Design review of the part built by this model. Coordinates are the model's own, in mm. A direction names the side the tool comes from. Coordinates: 2 decimals unless noted, no trailing zeros. Loops run counter-clockwise (first coordinate to the right, second up) from the corner with the lowest first, then second, coordinate; pieces in that order, holes last. Notation, with made-up numbers: M 84,75 L 107,75 A17 cw 107,82 Z; hole C 8,-19 d1. An arc over 180 degrees is marked long. Answer as CSV lines item,"result". Start each with the question number.
from build123d import *

# Parameters (mm, degrees)
SKETCH009_W             = 84
SKETCH009_H             = 70
PAD002_DEPTH            = 2
SKETCH010_W             = 2
SKETCH010_H             = 7
PAD003_DEPTH            = 2
SKETCH012_W             = 8
SKETCH012_H             = 6.8
PAD004_DEPTH            = 4
SKETCH013_W             = 7
SKETCH013_H             = 6
PAD005_DEPTH            = 4
SKETCH011_W             = 8
SKETCH011_H             = 6.8
PAD006_DEPTH            = 4
SKETCH014_R             = 1.15
POCKET002_DEPTH         = 81.001
SKETCH016_R             = 1.15
POCKET003_DEPTH         = 8.501
SKETCH018_W             = 11.5
SKETCH018_H             = 11.5
POCKET004_DEPTH         = 5
POCKET005_DEPTH         = 5
POCKET006_DEPTH         = 5
SKETCH021_W             = 1
SKETCH021_H             = 7
PAD007_DEPTH            = 1
SKETCH022_W             = 9
SKETCH022_H             = 10
POCKET007_DEPTH         = 0.4
FILLET_R                = 3
BODY002_PITCH_ANGLE     = -90
BODY002_PLACEMENT_ANGLE = 90
PAD001_DEPTH            = 35
SKETCH007_W             = 11.5
SKETCH007_H             = 11.5
POCKET001_DEPTH         = 13
FILLET001_R             = 3
SKETCH025_W             = 6.5
SKETCH025_H             = 9
SKETCH025_W_2           = 9
SKETCH025_H_2           = 6.5
POCKET008_DEPTH         = 8


with BuildPart() as back:
    # Sketch009 → Pad002 (new body)
    with BuildSketch(Plane.XY):
        Rectangle(SKETCH009_W, SKETCH009_H)
    extrude(amount=PAD002_DEPTH)

    # Sketch010 (on Face6 of Pad002) → Pad003 (join)
    with BuildSketch(Plane.XY.offset(2)):
        with Locations((-38, -1)):
            Rectangle(SKETCH010_W, SKETCH010_H)
        Polygon((-21, 32), (39, 32), (39, -4), (37, -4), (37, 30), (-21, 30), align=None)
    extrude(amount=PAD003_DEPTH)

    # Sketch012 (on Face15 of Pad003) → Pad004 (join)
    with BuildSketch(Plane.YZ.offset(39)):
        with Locations((0, 5.4)):
            Rectangle(SKETCH012_W, SKETCH012_H)
    extrude(amount=-PAD004_DEPTH)

    # Sketch013 (on Face9 of Pad004) → Pad005 (join)
    with BuildSketch(Plane(origin=(-39, 0, 0), x_dir=(0, -1, 0), z_dir=(-1, 0, 0))):
        with Locations((1, 5)):
            Rectangle(SKETCH013_W, SKETCH013_H)
    extrude(amount=-PAD005_DEPTH)

    # Sketch011 (on Face16 of Pad003) → Pad006 (join)
    with BuildSketch(Plane(origin=(0, 32, 0), x_dir=(-1, 0, 0), z_dir=(0, 1, 0))):
        with Locations((-29, 5.4)):
            Rectangle(SKETCH011_W, SKETCH011_H)
        with Locations((14, 5.4)):
            Rectangle(SKETCH011_W, SKETCH011_H)
    extrude(amount=-PAD006_DEPTH)

    # Sketch014 (on Face44 of Pad006) → Pocket002 (cut, through all)
    with BuildSketch(Plane.YZ.offset(39)):
        with Locations((0, 5)):
            Circle(SKETCH014_R)
    extrude(amount=-POCKET002_DEPTH, mode=Mode.SUBTRACT)

    # Sketch016 → Pocket003 (cut, through all)
    with BuildSketch(Plane.XZ.offset(-26.5)):
        with Locations((-13, 5)):
            Circle(SKETCH016_R)
        with Locations((30, 5)):
            Circle(SKETCH016_R)
    extrude(amount=-POCKET003_DEPTH, mode=Mode.SUBTRACT)

    # Sketch018 (on Face5 of Pocket003) → Pocket004 (cut)
    with BuildSketch(Plane.XY.offset(2)):
        with Locations((0, 17.75)):
            Rectangle(SKETCH018_W, SKETCH018_H)
    extrude(amount=-POCKET004_DEPTH, mode=Mode.SUBTRACT)

    # Sketch019 (on Face31 of Pocket004) → Pocket005 (cut)
    with BuildSketch(Plane.XZ.offset(-28)):
        Polygon((29.125944, 9.042901), (33.258869, 4.499726), (33.258869, 9.042901), align=None)
    extrude(amount=-POCKET005_DEPTH, mode=Mode.SUBTRACT)

    # Sketch020 (on Face36 of Pocket005) → Pocket006 (cut)
    with BuildSketch(Plane(origin=(35, 0, 0), x_dir=(0, -1, 0), z_dir=(-1, 0, 0))):
        Polygon((2.77547, 8.938441), (6.386171, 3.079567), (6.386171, 8.938441), align=None)
    extrude(amount=-POCKET006_DEPTH, mode=Mode.SUBTRACT)

    # Sketch021 (on Face40 of Pocket006) → Pad007 (join)
    with BuildSketch(Plane.XY.offset(8)):
        with Locations((-38.5, -1)):
            Rectangle(SKETCH021_W, SKETCH021_H)
    extrude(amount=PAD007_DEPTH)

    # Sketch022 (on Face5 of Pocket005) → Pocket007 (cut)
    with BuildSketch(Plane.XY.offset(2)):
        with Locations((-30.3, 30)):
            Rectangle(SKETCH022_W, SKETCH022_H)
    extrude(amount=-POCKET007_DEPTH, mode=Mode.SUBTRACT)

    # Fillet
    fillet_edges = [back.edges().sort_by_distance(p)[0] for p in [
        (42, 35, 1),
        (-42, 35, 1),
    ]]
    fillet(fillet_edges, radius=FILLET_R)


with BuildPart() as back_1:
    # Body002 pitch: moved
    add(back.part.rotate(Axis((0, 0, 0), (0, 1, 0)), BODY002_PITCH_ANGLE))


with BuildPart() as back_2:
    # Body002 placement: moved
    add(back_1.part.rotate(Axis((0, 0, 0), (0, 0, 1)), BODY002_PLACEMENT_ANGLE))


with BuildPart() as curve:
    # Sketch006 → Pad001 (new body, symmetric)
    with BuildSketch(Plane(origin=(0, 0, 0), x_dir=(0, 0, -1), z_dir=(1, 0, 0))):
        with BuildLine():
            ThreePointArc((-42, 3.4), (0, 0.674728), (42, 3.4))
            Line((42, -0.1), (42, 3.4))
            Line((-42, -0.1), (42, -0.1))
            Line((-42, 3.4), (-42, -0.1))
        make_face()
    extrude(amount=PAD001_DEPTH, both=True)

    # Sketch007 (on Face3 of Pad001) → Pocket001 (cut)
    with BuildSketch(Plane.XZ.offset(0.1)):
        with Locations((-17.75, 0)):
            Rectangle(SKETCH007_W, SKETCH007_H)
    extrude(amount=-POCKET001_DEPTH, mode=Mode.SUBTRACT)

    # Fillet001
    fillet001_edges = [curve.edges().sort_by_distance(p)[0] for p in [
        (-35, 1.65, -42),
        (-35, 1.65, 42),
    ]]
    fillet(fillet001_edges, radius=FILLET001_R)

    # Boolean: union Back
    add(back_2.part)

    # Sketch025 (on Face32 of Boolean) → Pocket008 (cut, symmetric)
    with BuildSketch(Plane.XZ.offset(2)):
        with Locations((-28.75, 0)):
            Rectangle(SKETCH025_W, SKETCH025_H)
        with Locations((-15.55, 13.625)):
            Rectangle(SKETCH025_W_2, SKETCH025_H_2)
        with Locations((-2.05, 0)):
            Rectangle(SKETCH025_W, SKETCH025_H)
        with Locations((-15.55, -13.625)):
            Rectangle(SKETCH025_W_2, SKETCH025_H_2)
    extrude(amount=POCKET008_DEPTH, both=True, mode=Mode.SUBTRACT)


solid = curve.part
Item 1: For pin 1 (10 mm diameter, centred on x = 23.5, z = 31.5, fed in from +Y); pin 2 (12 mm diameter, centred on x = 0, z = 17, fed in from +Y); pin 3 (8 mm diameter, centred on x = -12, z = 9.5, fed in from -Y), all flat-tipped, find the tip position at first contact; note any pin that passes through.
Item 2: For line 1 along Z through (x, y) = (-17.5, 0.5) (3 decimals); line 2 along X through (y, z) = (-5, -37.9); line 3 along Y through (x, z) = (22.5, 10), list the stretches that pass through material, from the lowest coordinate up. Write a range as from..to.
Item 3: For faces 1 (the face through (1.2, -1, 0)), 2 (the face through (-1, -6, 35)), 3 (the face through (-4, -6, 37)), 4 (the face through (-31, -4, -19)), list the 3-axis set-ups (+Z, -Z, +X, -X, +Y, -Y) from which the entire face can be reached by the end or side of a thin tool; tool diameter is ignored.
Item 4: Add section B-B (z = -13). Give the boundary of the cut face in (x, y).
Item 5: Add section D-D (x = 28.5). Give the boundary of the cut face in (y, z).
Item 6: Add section C-C (z = -1.5). Give the boundary of the cut face in (x, y).
Item 7: Add section A-A (x = 0). Give the boundary of the cut face in (y, z), plus the area to 3 significant figures.
Response:
1,pin 1,"y = 2.73"
1,pin 2,"y = 1.49"
1,pin 3,"y = -2"
2,line 1,"-42..-16.875, -10.375..-5.75, 5.75..10.375, 16.875..42"
2,line 2,"-2.5..-1.15, 1.15..4.5"
2,line 3,"-2..0.83"
3,face 1,"+Y, -Y"
3,face 2,"+X, -Y"
3,face 3,"-Z, -Y"
3,face 4,"-Z, +X, -X, -Y"
4,outline,"M -35,-2 L -32,-2 L -32,-3.85 L -28,-3.85 L -28,-2 L -20.05,-2 L -20.05,0.93 L -35,0.93 Z; M -32,-8.8 L -28,-8.8 L -28,-6.15 L -32,-6.15 Z; M -11.05,-2 L 35,-2 L 35,0.93 L -11.05,0.93 Z"
5,outline,"M -2,-42 L 3.4,-42 A325 cw 3.4,42 L -2,42 Z"
6,outline,"M -35,-2 L -32,-2 L -32,0.68 L -35,0.68 Z; M -25.5,-2 L -23.5,-2 L -23.5,0.68 L -25.5,0.68 Z; M -12,-2 L -5.3,-2 L -5.3,0.68 L -12,0.68 Z; M 1.2,-2 L 35,-2 L 35,0.68 L 1.2,0.68 Z"
7,outline,"M -9,-39 L -6.15,-39 L -6.15,-35 L -8,-35 L -8,-38 L -9,-38 Z; M -8.8,35 L -6.15,35 L -6.15,39 L -8.8,39 Z; M -3.85,-39 L -2,-39 L -2,-42 L 3.4,-42 A325 cw 0.71,-4.5 L -2,-4.5 L -2,-35 L -3.85,-35 Z; M -3.85,35 L -2,35 L -2,4.5 L 0.71,4.5 A325 cw 3.4,42 L -2,42 L -2,39 L -3.85,39 Z"
7,area,"310 mm²"
